from build123d import *

# Parameters (mm, degrees)
SKETCH1_W           = 30
SKETCH1_H           = 30
SKETCH1_R           = 2.15
BOSS_EXTRUDE1_DEPTH = 3.175
SKETCH2_W           = 30.005666414
SKETCH2_H           = 19.009049167
SKETCH2_W_2         = 23.655666414
SKETCH2_H_2         = 12.659049167
BOSS_EXTRUDE2_DEPTH = 15
SKETCH3_W           = 30.005666414
SKETCH3_H           = 19.009049167
BOSS_EXTRUDE3_DEPTH = 2
SKETCH4_W           = 15
SKETCH4_H           = 15
CUT_EXTRUDE1_DEPTH  = 31.005666414
FILLET1_R           = 2.5


with BuildPart() as part:
    # Sketch1 → Boss-Extrude1 (new body)
    with BuildSketch(Plane.XY):
        Rectangle(SKETCH1_W, SKETCH1_H)
        with Locations((-9.924911661, 9.924911661)):
            Circle(SKETCH1_R, mode=Mode.SUBTRACT)
        with Locations((9.924911661, 9.924911661)):
            Circle(SKETCH1_R, mode=Mode.SUBTRACT)
    extrude(amount=BOSS_EXTRUDE1_DEPTH)

    # Sketch2 → Boss-Extrude2 (add)
    with BuildSketch(Plane.XY.offset(3.175)):
        with Locations((0.002833207, -5.495475417)):
            Rectangle(SKETCH2_W, SKETCH2_H)
        with Locations((0.002833207, -5.495475417)):
            Rectangle(SKETCH2_W_2, SKETCH2_H_2, mode=Mode.SUBTRACT)
    extrude(amount=BOSS_EXTRUDE2_DEPTH)

    # Sketch3 → Boss-Extrude3 (add)
    with BuildSketch(Plane.XY.offset(18.175)):
        with Locations((0.002833207, -5.495475417)):
            Rectangle(SKETCH3_W, SKETCH3_H)
    extrude(amount=BOSS_EXTRUDE3_DEPTH)

    # Sketch4 → Cut-Extrude1 (cut, through all)
    with BuildSketch(Plane.ZY.offset(15)):
        with Locations((10.675, -5.5)):
            Rectangle(SKETCH4_W, SKETCH4_H)
    extrude(amount=-CUT_EXTRUDE1_DEPTH, mode=Mode.SUBTRACT)

    # Fillet1
    fillet1_edges = [part.edges().sort_by_distance(p)[0] for p in [
        (0, 4.009049167, 3.175),
        (0.002833207, -15, 20.175),
        (0.002833207, 4.009049167, 20.175),
        (0, -13, 3.175),
        (0, 2, 3.175),
        (0.002833207, 2, 18.175),
        (0.002833207, -13, 18.175),
    ]]
    fillet(fillet1_edges, radius=FILLET1_R)


solid = part.part
Can you work these out from the model? Positions are in its coordinate system, mm. A direction names the side the tool comes from. Round coordinates to 2 decimals unless told otherwise and drop trailing zeros. Write each loop counter-clockwise with the first axis right and the second up, starting at its lowest first coordinate (ties: lowest second). Pieces come first, ordered by that corner, then holes. Notation, with made-up numbers: M 75.25,75 L 104.25,75 A18 cw 104.25,93 Z; hole C -15,-0.5 d5. An arc over 180 degrees is marked long. Use a Markdown table: item, result.
Item 1: For pin 1 Ø10 at (x, z) = (-6, 11) entering from +Y; pin 2 Ø5 at (y, z) = (-2, 4) entering from +X; pin 3 Ø8 at (x, y) = (-10.5, 8.5) entering from +Z, each with a flat end and sliding along its axis, tell me the tip position at first contact or that it passes through.
Found:
| item | result |
|---|---|
| pin 1 | stops at y = 4.01 |
| pin 2 | stops at x = 15 |
| pin 3 | stops at z = 4.19 |
Item 2: I want a section at D-D (z = 8.75). List the corners of the cut face in (x, y) for me, and give its area (3 significant figures).
Found:
| item | result |
|---|---|
| outline | M -15,-15 L 15.01,-15 L 15.01,-13 L -15,-13 Z; M -15,2 L 15.01,2 L 15.01,4.01 L -15,4.01 Z |
| area | 120 mm2 |
Item 3: I want a section at C-C (x = 11). List the corners of the cut face in (y, z) for me (3 decimals).
Found:
| item | result |
|---|---|
| outline | M -15,0 L 8.063,0 L 8.063,3.175 L 6.509,3.175 A2.5 cw 4.009,5.675 L 4.009,17.675 A2.5 ccw 1.509,20.175 L -12.5,20.175 A2.5 ccw -15,17.675 Z; M 11.787,0 L 15,0 L 15,3.175 L 11.787,3.175 Z; hole M -13,5.675 A2.5 ccw -10.5,3.175 L -0.5,3.175 A2.5 ccw 2,5.675 L 2,15.675 A2.5 ccw -0.5,18.175 L -10.5,18.175 A2.5 ccw -13,15.675 Z |
Item 4: If I drill on line 1 along Y through (x, z) = (-13, 12); line 2 along Z through (x, y) = (-3.5, -8) (3 decimals); line 3 along X through (y, z) = (14.5, 2.25), over which ranges is the centre line in solid material (lowest first)? Write a range as [from, to].
Found:
| item | result |
|---|---|
| line 1 | y = [-15, -13], [2, 4.01] |
| line 2 | z = [0, 3.175], [18.175, 20.175] |
| line 3 | x = [-15, 15] |
Item 5: I want a section at B-B (x = -1.5). List the corners of the cut face in (y, z) for me (3 decimals), and give its area (3 significant figures).
Found:
| item | result |
|---|---|
| outline | M -15,0 L 15,0 L 15,3.175 L 6.509,3.175 A2.5 cw 4.009,5.675 L 4.009,17.675 A2.5 ccw 1.509,20.175 L -12.5,20.175 A2.5 ccw -15,17.675 Z; hole M -13,5.675 A2.5 ccw -10.5,3.175 L -0.5,3.175 A2.5 ccw 2,5.675 L 2,15.675 A2.5 ccw -0.5,18.175 L -10.5,18.175 A2.5 ccw -13,15.675 Z |
| area | 197 mm2 |
Item 6: Which directions (+Z, -Z, +X, -X, +Y, -Y) give clear straight access to the entire face, cutting with the end or side of a thin tool? Please do faces 1 (the face through (0, 4.009, 12)), 2 (the face through (0, -6, 18.175)).
Found:
| item | result |
|---|---|
| face 1 | +Z, +X, -X, +Y |
| face 2 | +X, -X |
Item 7: We'd pull the mould along Y, two halves only. Please class faces 3 (the face through (0, 0, 0)), 4 (the face through (0.21, 4.72, 3.93)), 5 (the face through (0.21, -12.29, 17.42)): released by +Y, released by -Y, zero draft, split by the parting line, or undercut.
Found:
| item | result |
|---|---|
| face 3 | zero draft |
| face 4 | released by +Y |
| face 5 | undercut |
Item 8: I want a section at A-A (y = -2.5). List the corners of the cut face in (x, z) for me (3 decimals).
Found:
| item | result |
|---|---|
| outline | M -15,0 L 15,0 L 15,3.175 L -15,3.175 Z; M -15,18.175 L 15.006,18.175 L 15.006,20.175 L -15,20.175 Z |
